from build123d import *

# Parameters (mm, degrees)
SALIENTE_EXTRUIR1_DEPTH = 175
REDONDEO1_R             = 5


with BuildPart() as part:
    # Croquis1 → Saliente-Extruir1 (new, symmetric)
    with BuildSketch(Plane(origin=(0, 0, 0), x_dir=(0, 0, -1), z_dir=(1, 0, 0))):
        Polygon((-21.789612973, 0), (-21.789612973, 15), (-10, 15), (-10, 75), (10, 75), (10, -75), (-10, -75), (-10, -15), (-21.789612973, -15), align=None)
    extrude(amount=SALIENTE_EXTRUIR1_DEPTH, both=True)

    # Redondeo1
    redondeo1_edges = [part.edges().sort_by_distance(p)[0] for p in [
        (-175, -45, 10),
        (-175, -15, 15.894806486),
        (-175, 15, 15.894806486),
        (-175, 45, 10),
        (0, 75, 10),
        (0, -75, 10),
        (0, -15, 10),
        (0, 15, 10),
        (175, -15, 15.894806486),
        (175, -45, 10),
        (175, 45, 10),
        (175, 15, 15.894806486),
    ]]
    fillet(redondeo1_edges, radius=REDONDEO1_R)


solid = part.part
The listing builds one solid part. Answer for the finished solid, in the listing's coordinates (mm). A direction names the side the tool comes from. Round coordinates to 2 decimals unless told otherwise and drop trailing zeros. Order: outer loops, then holes, each group sorted by start corner. A loop starts at its lowest first (then second) coordinate and runs counter-clockwise, first axis right, second up. Notation, with made-up numbers: (-20.75, 21.25) - (8.25, 21.25) arc R29 cw to (8.25, 58.25) - close; hole circle Ø4 at (55, 45). An arc over 180 degrees is marked (long way). Write item = value, one per line. Start each with the question number.
1) For faces 1 (the flat face through (2, -15, 18)), 2 (the flat face through (2, 0, 21.79)), 3 (the flat face through (2, 45, 10)), determine the directions among +Z, -Z, +X, -X, +Y, -Y from which every point of the face is accessible in a straight line to the end or side of a thin tool.
2) Section A-A, the plane x = -109.5 is taken. Write down the section's boundary in (y, z), plus the area to 3 significant figures.
3) Given pin 1 (1.5 mm diameter, centred on x = -134.5, z = 18.5, fed in from -Y); pin 2 (7.5 mm diameter, centred on x = -27, z = 17, fed in from +Y); pin 3 (7.5 mm diameter, centred on x = -31.5, z = 17.5, fed in from -Y), each flat-ended and moving along its own axis, determine where each tip first touches the part or whether it passes through.
4) Section B-B, the plane y = -31.5 is taken. Write down the section's boundary in (x, z).
5) Straight lines are drawn through the part: L1, parallel to Z at x = -157, y = 63; L2, parallel to Y at x = -118, z = 16; L3, parallel to Y at x = -116.5, z = 11.5. For each, find the intervals that lie inside material, in ascending order.
Results list:
q1.face_1 = +Z, +X, -X, -Y
q1.face_2 = +Z, +X, -X, +Y, -Y
q1.face_3 = +Z, +X, -X, +Y
q2.outline = (-75, -10) - (75, -10) - (75, 5) arc R5 ccw to (70, 10) - (20, 10) arc R5 cw to (15, 15) - (15, 21.79) - (-15, 21.79) - (-15, 15) arc R5 cw to (-20, 10) - (-70, 10) arc R5 ccw to (-75, 5) - close
q2.area = 3,350 mm^2
q3.pin_1 = -15
q3.pin_2 = 15.32
q3.pin_3 = -15.16
q4.outline = (-175, -10) - (175, -10) - (175, 5) arc R5 ccw to (170, 10) - (-170, 10) arc R5 ccw to (-175, 5) - close
q5.L1 = -10 to 10
q5.L2 = -15 to 15
q5.L3 = -16.43 to 16.43
